Design review of the part built by this model. Coordinates are the model's own, in mm. Face numbers are marked on the shaded views. Coordinates: 2 decimals unless noted, no trailing zeros. Loops run counter-clockwise (first coordinate to the right, second up) from the corner with the lowest first, then second, coordinate; pieces in that order, holes last.
Q1. Draft analysis for pull direction Y (two halves, no side actions). For the marked faces 1 and 2, state which applies: released by +Y, released by -Y, zero draft, split by the parting line, or undercut.
Q2. For P1, Ø5, axis at x = -7, y = 1.5, coming from the +Z side, flat-tipped, find the tip position at first contact; note if it passes through.
Q3. Add section A-A on x = -7. Give the boundary of the cut face in (y, z), and give its area (3 significant figures).
Q4. Wall thickness on probe 1 along Y at (x, z) = (-13, 1.7); probe 2 along Y at (x, z) = (-10.5, 0.3); probe 3 along Z at (x, y) = (-21.5, -1.25): over which ranges is each line inside the solid? List them lowest first.
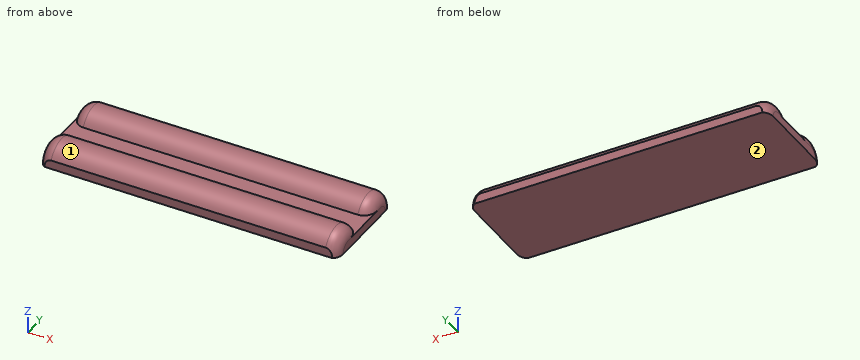
```python
from build123d import *

# Parameters (mm, degrees)
F0_W     = 50
F0_H     = 16
F1_DEPTH = 1.5
F3_DEPTH = 50
F4_R     = 1.99999


# Not quite as in the source:
# - a fillet or chamfer is up to 0.001 mm smaller than in the source, because OpenCascade refuses the exact size


with BuildPart() as f1:
    # F0 (on Top) → F1 (new body)
    with BuildSketch(Plane.XY):
        Rectangle(F0_W, F0_H)
    extrude(amount=-F1_DEPTH)

    # F2 (on face) → F3 (join)
    with BuildSketch(Plane(origin=(-25, 0, 0), x_dir=(0, -1, 0), z_dir=(-1, 0, 0))):
        with BuildLine():
            ThreePointArc((-1.6754446797, 0), (-4.8377223398, 2), (-8, 0))
            Line((-8, 0), (-1.6754446797, 0))
        make_face()
        with BuildLine():
            ThreePointArc((8, 0), (4.8377223398, 2), (1.6754446797, 0))
            Line((1.6754446797, 0), (8, 0))
        make_face()
    extrude(amount=-F3_DEPTH)

    # F4 (radius 2 in the source; OpenCascade refuses exactly that, so slightly less here)
    f4_edges = [f1.edges().sort_by_distance(p)[0] for p in [
        (-25, -4.837722, 2),
        (-25, 4.837722, 2),
        (25, -4.837722, 2),
        (25, 4.837722, 2),
    ]]
    fillet(f4_edges, radius=F4_R)


solid = f1.part
```
Entries:
1. face 1: undercut
1. face 2: zero draft
2. P1: stops at z = 1.9
3. outline: (-8, -1.5) - (8, -1.5) - (8, 0) arc R3.5 ccw to (1.68, 0) - (-1.68, 0) arc R3.5 ccw to (-8, 0) - close
3. area: 42.1 mm2
4. probe 1: y = -6.26 to -3.42, 3.42 to 6.26
4. probe 2: y = -7.84 to -1.84, 1.84 to 7.84
4. probe 3: z = -1.5 to 0
